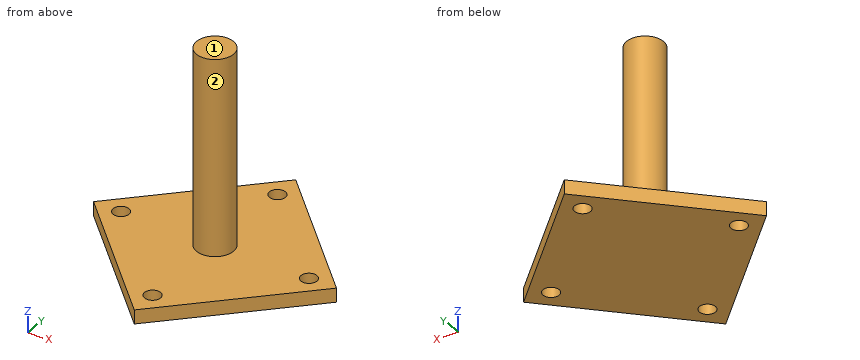
from build123d import *

# Parameters (mm, degrees)
SKETCH_1_R          = 2.65
EXTRUDE_1_DEPTH     = 30
SKETCH_2_W          = 35
SKETCH_2_H          = 35
EXTRUDE_2_DEPTH     = 2
SKETCH_8_R          = 1.15
CUT_EXTRUDE_5_DEPTH = 5
SKETCH_10_OUTSIDE_W = 48.576
SKETCH_10_OUTSIDE_H = 48.576
CUT_EXTRUDE_6_DEPTH = 5


with BuildPart() as part:
    # 스케치1 → 보스-돌출1 (new body)
    with BuildSketch(Plane.XY):
        Circle(SKETCH_1_R)
    extrude(amount=EXTRUDE_1_DEPTH)

    # 스케치2 → 보스-돌출2 (add)
    with BuildSketch(Plane(origin=(0, 0, 0), x_dir=(-1, 0, 0), z_dir=(0, 0, -1))):
        Rectangle(SKETCH_2_W, SKETCH_2_H)
    extrude(amount=-EXTRUDE_2_DEPTH)

    # 스케치8 → 컷-돌출5 (cut)
    with BuildSketch(Plane(origin=(0, 0, 0), x_dir=(-1, 0, 0), z_dir=(0, 0, -1))):
        with Locations((13.533711803, 0)):
            Circle(SKETCH_8_R)
        with Locations((0, -13.533711803)):
            Circle(SKETCH_8_R)
        with Locations((-13.533711803, 0)):
            Circle(SKETCH_8_R)
        with Locations((0, 13.533711803)):
            Circle(SKETCH_8_R)
    extrude(amount=-CUT_EXTRUDE_5_DEPTH, mode=Mode.SUBTRACT)

    # 스케치10 outside → 컷-돌출6 (cut)
    with BuildSketch(Plane.XY.offset(2)):
        Rectangle(SKETCH_10_OUTSIDE_W, SKETCH_10_OUTSIDE_H)
        Polygon((-17.5, 0), (0, 17.5), (17.5, 0), (0, -17.5), align=None, mode=Mode.SUBTRACT)
    extrude(amount=-CUT_EXTRUDE_6_DEPTH, mode=Mode.SUBTRACT)


solid = part.part
Geometry: final body of the model. Coordinates: model frame, mm. Face numbers are marked on the shaded views. A direction names the side the tool comes from. Round coordinates to 2 decimals unless told otherwise and drop trailing zeros. Loops run counter-clockwise (first coordinate to the right, second up) from the corner with the lowest first, then second, coordinate; pieces in that order, holes last.
Q1. Section A-A on y = -8. Return loops of the section in (x, z), plus the area to 3 significant figures.
Q2. Section B-B on z = 22.5. Return loops of the section in (x, y), plus the area to 3 significant figures.
Q3. Material intervals for L1, parallel to Z at x = -14, y = -2; L2, parallel to Y at x = 1, z = 16, sorted ascending.
Q4. Pin query (flat end, axial travel): P1, Ø3.5, axis at x = 0, y = -13.53, coming from the +Z side; P2, Ø6, axis at x = 0, z = 26.5, coming from the -Y side. Return the tip coordinate at first contact, or that it passes through.
Q5. Access query for the marked faces 1 and 2. Directions: +Z, -Z, +X, -X, +Y, -Y. A direction counts if a zero-diameter tool reaches every point of the face in a straight line with its end or side. Return the directions, or none.
Evaluation:
1. outline: (-9.5, 0) - (9.5, 0) - (9.5, 2) - (-9.5, 2) - close
1. area: 38.0 mm2
2. outline: circle Ø5.3 at (0, 0)
2. area: 22.1 mm2
3. L1: z = 0 to 2
3. L2: y = -2.45 to 2.45
4. P1: stops at z = 2
4. P2: stops at y = -2.65
5. face 1: +Z, +X, -X, +Y, -Y
5. face 2: +Z
